from build123d import *

# Parameters (mm, degrees)
F1_DEPTH = 15
F2_R     = 14.76375
F2_R_2   = 12.875
F3_DEPTH = 2.5
F5_D     = 11.50874


with BuildPart() as f1:
    # F0 (on Right) → F1 (new body)
    with BuildSketch(Plane.YZ):
        with BuildLine():
            Line((-175, -20), (0, -20))
            ThreePointArc((0, -20), (20, 0), (0, 20))
            Line((0, 20), (-175, 20))
            ThreePointArc((-175, 20), (-195, 0), (-175, -20))
        make_face()
        with BuildLine():
            ThreePointArc((-11.7637353516, 2.3695000693), (-8.4852813742, 8.4852813742), (-2.3695000693, 11.7637353516))
            ThreePointArc((-2.3695000693, 11.7637353516), (0, 9.61875), (2.3695000693, 11.7637353516))
            ThreePointArc((2.3695000693, 11.7637353516), (8.4852813742, 8.4852813742), (11.7637353516, 2.3695000693))
            ThreePointArc((11.7637353516, 2.3695000693), (9.61875, 0), (11.7637353516, -2.3695000693))
            ThreePointArc((11.7637353516, -2.3695000693), (8.4852813742, -8.4852813742), (2.3695000693, -11.7637353516))
            ThreePointArc((2.3695000693, -11.7637353516), (0, -9.61875), (-2.3695000693, -11.7637353516))
            ThreePointArc((-2.3695000693, -11.7637353516), (-8.4852813742, -8.4852813742), (-11.7637353516, -2.3695000693))
            ThreePointArc((-11.7637353516, -2.3695000693), (-9.61875, 0), (-11.7637353516, 2.3695000693))
        make_face(mode=Mode.SUBTRACT)
    extrude(amount=F1_DEPTH)

    # F2 (on face) → F3 (join)
    with BuildSketch(Plane.YZ.offset(15)):
        Circle(F2_R)
        Circle(F2_R_2, mode=Mode.SUBTRACT)
    extrude(amount=F3_DEPTH)

    # F5 (through all)
    with Locations(Plane.YZ.offset(15)):
        with Locations((-175, 0)):
            Hole(F5_D / 2)


solid = f1.part
Can you work these out from the model? Positions are in its coordinate system, mm. A direction names the side the tool comes from. Give positions to 0.01 mm unless a question says otherwise; leave off trailing zeros. Loops run counter-clockwise (first coordinate to the right, second up) from the corner with the lowest first, then second, coordinate; pieces in that order, holes last. Notation, with made-up numbers: (25, 62.25) - (29, 62.25) arc R26 cw to (29, 87.25) - close; hole circle Ø7 at (17.25, -20). An arc over 180 degrees is marked (long way). Return JSON: item names as keys, results as strings.
1. I'm going to push flat-ended pins straight in: pin 1 Ø1.5 at (y, z) = (-32.5, 5) entering from -X; pin 2 Ø12 at (y, z) = (-92.5, -3.5) entering from +X; pin 3 Ø10 at (x, z) = (3, -15) entering from +Y. Where does each tip first touch, or does it pass through?
Output values:
{"pin 1": "stops at x = 0", "pin 2": "stops at x = 15", "pin 3": "stops at y = 17.32"}
2. For faces 1 (the face through (7, 20, 0)), 2 (the face through (15, 0, 11)), which set-ups out of +Z, -Z, +X, -X, +Y, -Y let a thin tool reach every point of the face, with its end or its side?
Output values:
{"face 1": "+X, -X, +Y", "face 2": "+X"}
3. I want a section at B-B on z = 0. Please give me the cut outline in (x, y) (3 decimals), and give its area (3 significant figures).
Output values:
{"outline": "(0, -195) - (15, -195) - (15, -180.754) - (0, -180.754) - close; (0, -169.246) - (15, -169.246) - (15, -14.764) - (17.5, -14.764) - (17.5, -12.875) - (15, -12.875) - (15, -9.619) - (0, -9.619) - close; (0, 9.619) - (15, 9.619) - (15, 12.875) - (17.5, 12.875) - (17.5, 14.764) - (15, 14.764) - (15, 20) - (0, 20) - close", "area": "2,770 mm²"}
4. We'd pull the mould along Z, two halves only. Please class faces 3 (the face through (17.5, 1, 13)), 4 (the face through (7.4, -9.62, -0.05)), 5 (the face through (7, -89, -20)), 6 (the face through (7, -86, 20)): +Z half, -Z half, draft (parallel to the pull), parting line (faces both ways), or undercut.
Output values:
{"face 3": "draft", "face 4": "undercut", "face 5": "-Z half", "face 6": "+Z half"}
5. I want a section at C-C on y = -143. Please give me the cut outline in (x, z), and give its area (3 significant figures).
Output values:
{"outline": "(0, -20) - (15, -20) - (15, 20) - (0, 20) - close", "area": "600 mm²"}
6. I want a section at A-A on x = 10.25. Please give me the cut outline in (y, z), and give its area (3 significant figures).
Output values:
{"outline": "(-175, -20) - (0, -20) arc R20 ccw to (0, 20) - (-175, 20) arc R20 ccw to start; hole circle Ø11.51 at (-175, 0); hole (-11.76, -2.37) arc R12 ccw to (-2.37, -11.76) arc R2.38 cw to (2.37, -11.76) arc R12 ccw to (11.76, -2.37) arc R2.38 cw to (11.76, 2.37) arc R12 ccw to (2.37, 11.76) arc R2.38 cw to (-2.37, 11.76) arc R12 ccw to (-11.76, 2.37) arc R2.38 cw to start", "area": "7,730 mm²"}
7. If I drill on line 1 (Z direction, x = 15.65, y = 0) (3 decimals); line 2 (Y direction, x = 2.5, z = 10.5); line 3 (Z direction, x = 10, y = -175), over which ranges is the centre line in solid material (lowest first)?
Output values:
{"line 1": "z = -14.764 to -12.875, 12.875 to 14.764", "line 2": "y = -192.02 to -5.81, -1.85 to 1.85, 5.81 to 17.02", "line 3": "z = -20 to -5.75, 5.75 to 20"}
